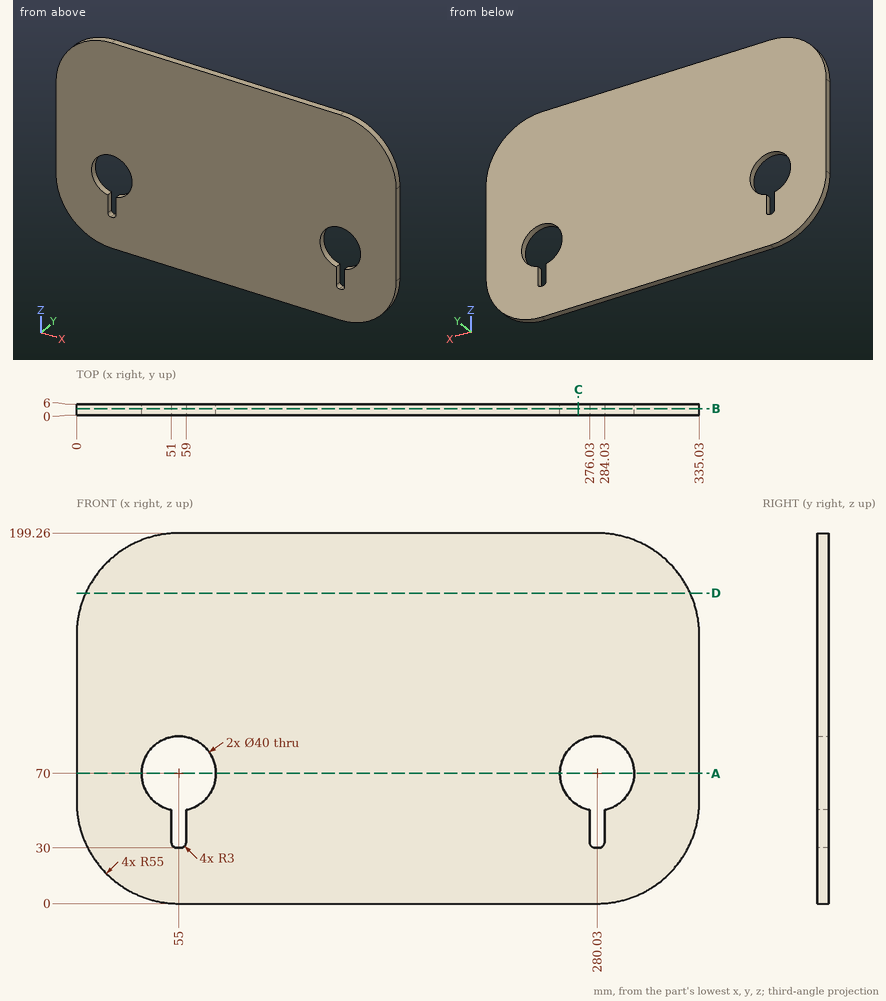
Input: dimensioned drawing with shaded views. Units: mm. Origin: part minimum x, y, z. Give positions to 0.01 mm unless a question says otherwise; leave off trailing zeros. Write each loop counter-clockwise with the first axis right and the second up, starting at its lowest first coordinate (ties: lowest second). Pieces come first, ordered by that corner, then holes. Notation, with made-up numbers: M 50.25,28 L 80.25,28 A24 ccw 80.25,61 Z; hole C 15.5,7.25 d7. An arc over 180 degrees is marked long. Return JSON: item names as keys, results as strings. Group by question number.
1) Cut plane D-D, the plane z = 167. Output: boundary loops of the cut face in (x, y), plus the area to 3 significant figures.
2) Cut plane A-A, the plane z = 70. Output: boundary loops of the cut face in (x, y).
3) Pin query (flat end, axial travel): P1, Ø1.8, axis at y = 4, z = 43, coming from the +X side; P2, Ø3, axis at y = 2.5, z = 45, coming from the -X side; P3, Ø1.5, axis at y = 5, z = 163, coming from the -X side. Return the tip coordinate at first contact, or that it passes through.
4) Material intervals for line 1 along X through (y, z) = (2.45, 70); line 2 along Z through (x, y) = (279.5, 1.2); line 3 along Z through (x, y) = (37, 2), sorted ascending. Write a range as [from, to].
5) Cut plane C-C, the plane x = 270. Output: boundary loops of the cut face in (y, z), plus the area to 3 significant figures.
6) Cut plane B-B, the plane y = 3.45. Output: boundary loops of the cut face in (x, z).
Recorded:
{
 "1": {"outline": "M 4.92,0 L 330.11,0 L 330.11,6 L 4.92,6 Z", "area": "1,950 mm²"},
 "2": {"outline": "M 0,0 L 35,0 L 35,6 L 0,6 Z; M 75,0 L 260.03,0 L 260.03,6 L 75,6 Z; M 300.03,0 L 335.03,0 L 335.03,6 L 300.03,6 Z"},
 "3": {"P1": "stops at x = 333.9", "P2": "stops at x = 0.66", "P3": "stops at x = 3.03"},
 "4": {"line 1": "x = [0, 35], [75, 260.03], [300.03, 335.03]", "line 2": "z = [0, 30], [89.99, 199.26]", "line 3": "z = [3.03, 61.28], [78.72, 196.23]"},
 "5": {"outline": "M 0,0 L 6,0 L 6,52.7 L 0,52.7 Z; M 0,87.3 L 6,87.3 L 6,199.26 L 0,199.26 Z", "area": "988 mm²"},
 "6": {"outline": "M 0,55 A55 ccw 55,0 L 280.03,0 A55 ccw 335.03,55 L 335.03,144.26 A55 ccw 280.03,199.26 L 55,199.26 A55 ccw 0,144.26 Z; hole M 51,33 A3 ccw 54,30 L 56,30 A3 ccw 59,33 L 59,50.4 A20 ccw long 51,50.4 Z; hole M 276.03,33 A3 ccw 279.03,30 L 281.03,30 A3 ccw 284.03,33 L 284.03,50.4 A20 ccw long 276.03,50.4 Z"}
}
